```python
from build123d import *

# Parameters (mm, degrees)
BOSS_EXTRU_1_DEPTH      = 5
ESQUISSE2_W             = 5
ESQUISSE2_H             = 10
ENL_V_MAT_EXTRU_1_DEPTH = 10
ENL_V_MAT_EXTRU_2_DEPTH = 10


with BuildPart() as part:
    # Esquisse1 → Boss.-Extru.1 (new body)
    with BuildSketch(Plane.XY):
        Polygon((-80, 0), (-40, 40), (-30, 40), (-30, 35), (70, 35), (70, 40), (80, 40), (80, -40), (70, -40), (70, -45), (-70, -45), (-70, -40), (-80, -40), (-80, -35), (-75, -35), (-75, -25), (-80, -25), (-80, -15), (-75, -15), (-75, -5), (-80, -5), align=None)
    extrude(amount=BOSS_EXTRU_1_DEPTH)

    # Esquisse2 → Enlèv. mat.-Extru.1 (cut)
    with BuildSketch(Plane.XY.offset(5)):
        with Locations((77.5, -30)):
            Rectangle(ESQUISSE2_W, ESQUISSE2_H)
        with Locations((77.5, -10)):
            Rectangle(ESQUISSE2_W, ESQUISSE2_H)
        with Locations((77.5, 10)):
            Rectangle(ESQUISSE2_W, ESQUISSE2_H)
        with Locations((77.5, 30)):
            Rectangle(ESQUISSE2_W, ESQUISSE2_H)
    extrude(amount=-ENL_V_MAT_EXTRU_1_DEPTH, mode=Mode.SUBTRACT)

    # Esquisse3 → Enlèv. mat.-Extru.2 (cut)
    with BuildSketch(Plane.XY.offset(5)):
        Polygon((-43.535533906, 36.464466094), (-54.142135624, 25.857864376), (-50.606601718, 22.32233047), (-40, 32.928932188), align=None)
        Polygon((-65.857864376, 14.142135624), (-76.464466094, 3.535533906), (-72.928932188, 0), (-62.32233047, 10.606601718), align=None)
    extrude(amount=-ENL_V_MAT_EXTRU_2_DEPTH, mode=Mode.SUBTRACT)


solid = part.part
```
Geometry check sheet. Reference: the model listing, model coordinates, mm. A direction names the side the tool comes from. Round coordinates to 2 decimals unless told otherwise and drop trailing zeros. Order: outer loops, then holes, each group sorted by start corner. A loop starts at its lowest first (then second) coordinate and runs counter-clockwise, first axis right, second up. Notation, with made-up numbers: M 22,31.25 L 68,31.25 A26 cw 68,66.25 Z; hole C -37,6 d3. An arc over 180 degrees is marked long. Write item = value, one per line.
Q1. Scan lines: line 1 (Y direction, x = 29.5, z = 0.7); line 2 (X direction, y = -31, z = 1.2); line 3 (X direction, y = 24, z = 4). Record each from-to range of solid material in increasing order.
Answer block:
line_1 = -45 to 35
line_2 = -75 to 75
line_3 = -56 to -52.28, -48.93 to 80
Q2. Release check for a two-part mould opening along Y. For faces 5 (the flat face through (-30, 38, 2)), 6 (the flat face through (75, 40, 2)), 7 (the flat face through (-78, -15, 2)) record: released by +Y, released by -Y, zero draft, split by the parting line, or undercut.
Answer block:
face_5 = zero draft
face_6 = released by +Y
face_7 = undercut
Q3. Section check B-B (y = -32). Enter the section's corners in (x, z), plus the area to 3 significant figures.
Answer block:
outline = M -75,0 L 75,0 L 75,5 L -75,5 Z
area = 750 mm^2
Q4. Set-up check for faces 1 (the flat face through (-75, -40, 2)), 2 (the flat face through (75, -40, 2)), 3 (the flat face through (77, -35, 3)), 4 (the flat face through (70, 37, 2)): record each of +Z, -Z, +X, -X, +Y, -Y from which the full face is reachable in a straight line by a thin tool's end or side.
Answer block:
face_1 = +Z, -Z, -X, -Y
face_2 = +Z, -Z, +X, -Y
face_3 = +Z, -Z, +X
face_4 = +Z, -Z, +Y
Q5. Depth check by flat-ended pin: pin 1 Ø1.5 at (y, z) = (24, 0.5) entering from -X; pin 2 Ø1.5 at (x, y) = (-55, 27) entering from +Z (3 decimals); pin 3 Ø1.5 at (x, z) = (78, 1.5) entering from -Y; pin 4 Ø1.5 at (y, z) = (12, 2.5) entering from +X. Enter the tip coordinate at first touch or a pass-through.
Answer block:
pin_1 = -56.75
pin_2 = through
pin_3 = -40
pin_4 = 75
Q6. Section check A-A (x = 60.5). Enter the section's corners in (y, z), plus the area to 3 significant figures.
Answer block:
outline = M -45,0 L 35,0 L 35,5 L -45,5 Z
area = 400 mm^2
